```python
from build123d import *

# Parameters (mm, degrees)
F1_DEPTH  = 6
F2_R      = 27.5
F3_DEPTH  = 30
F4_R      = 14
F5_DEPTH  = 40
F6_W      = 56
F6_H      = 10
F7_DEPTH  = 8
F8_R      = 3
F9_DEPTH  = 10.5
F10_W     = 56
F10_H     = 66
F11_DEPTH = 25
F12_SIZE  = 5
F14_DEPTH = 30


with BuildPart() as f1:
    # F0 (on Front) → F1 (new body)
    with BuildSketch(Plane.XZ):
        with BuildLine():
            ThreePointArc((38, 33), (35.0710678119, 40.0710678119), (28, 43))
            Line((28, 43), (-28, 43))
            ThreePointArc((-28, 43), (-35.0710678119, 40.0710678119), (-38, 33))
            Line((-38, 33), (-38, -33))
            ThreePointArc((-38, -33), (-35.0710678119, -40.0710678119), (-28, -43))
            Line((-28, -43), (28, -43))
            ThreePointArc((28, -43), (35.0710678119, -40.0710678119), (38, -33))
            Line((38, -33), (38, 33))
        make_face()
    extrude(amount=F1_DEPTH)

    # F2 (on face) → F3 (join)
    with BuildSketch(Plane(origin=(0, 0, 0), x_dir=(-1, 0, 0), z_dir=(0, 1, 0))):
        Circle(F2_R)
    extrude(amount=F3_DEPTH)

    # F4 (on face) → F5 (join)
    with BuildSketch(Plane(origin=(0, 30, 0), x_dir=(-1, 0, 0), z_dir=(0, 1, 0))):
        Circle(F4_R)
    extrude(amount=F5_DEPTH)

    # F6 (on face) → F7 (join)
    with BuildSketch(Plane.XZ.offset(6)):
        with Locations((0, -38)):
            Rectangle(F6_W, F6_H)
    extrude(amount=F7_DEPTH)

    # F8 (on face) → F9 (join)
    with BuildSketch(Plane(origin=(0, 0, -43), x_dir=(1, 0, 0), z_dir=(0, 0, -1))):
        with Locations((-20, 10.148444213)):
            Circle(F8_R)
        with Locations((20, 10.148444213)):
            Circle(F8_R)
    extrude(amount=F9_DEPTH)

    # F10 (on face) → F11 (join)
    with BuildSketch(Plane.XZ.offset(6)):
        Rectangle(F10_W, F10_H)
    extrude(amount=F11_DEPTH)

    # F12
    f12_edges = [f1.edges().sort_by_distance(p)[0] for p in [
        (0, -31, 33),
        (28, -31, 0),
        (-28, -31, 0),
        (-28, -18.5, 33),
        (28, -18.5, 33),
        (28, -22.5, -33),
        (0, -31, -33),
        (-28, -22.5, -33),
        (0, -6, 43),
    ]]
    chamfer(f12_edges, length=F12_SIZE)

    # F13 (on face) → F14 (cut, through all)
    with BuildSketch(Plane(origin=(0, 30, 0), x_dir=(-1, 0, 0), z_dir=(0, 1, 0))):
        with BuildLine():
            Line((-17.7552809046, 21), (17.7552809046, 21))
            ThreePointArc((17.7552809046, 21), (0, 27.5), (-17.7552809046, 21))
        make_face()
        with BuildLine():
            ThreePointArc((27.5, 0), (25.8239230172, 9.4538352006), (21, 17.7552809046))
            Line((21, 17.7552809046), (21, -17.7552809046))
            ThreePointArc((21, -17.7552809046), (25.8239230172, -9.4538352006), (27.5, 0))
        make_face()
        with BuildLine():
            ThreePointArc((-17.7552809046, -21), (0, -27.5), (17.7552809046, -21))
            Line((17.7552809046, -21), (-17.7552809046, -21))
        make_face()
        with BuildLine():
            Line((-21, -17.7552809046), (-21, 17.7552809046))
            ThreePointArc((-21, 17.7552809046), (-27.5, 0), (-21, -17.7552809046))
        make_face()
    extrude(amount=-F14_DEPTH, mode=Mode.SUBTRACT)


solid = f1.part
```
Can you work these out from the model? Positions are in its coordinate system, mm. A direction names the side the tool comes from. Give positions to 0.01 mm unless a question says otherwise; leave off trailing zeros. Order: outer loops, then holes, each group sorted by start corner. A loop starts at its lowest first (then second) coordinate and runs counter-clockwise, first axis right, second up. Notation, with made-up numbers: (3, 74) - (35, 74) arc R23 ccw to (35, 108) - close; hole circle Ø3 at (42.5, 37.5). An arc over 180 degrees is marked (long way). Use a Markdown table: item, result. Add a question column.
Q1. If we mould it in two halves opening along X, with no side actions, what happens to faces 6 (the flat face through (-24.5, -27.6, -29.9)), 7 (the flat face through (25, -20, -31)), 8 (the cylindrical face through (-22.21, -12.18, -48.18)), 9 (the flat face through (0, 15, -21))? For each: released by +X, released by -X, zero draft, split by the parting line, or undercut.
Q2. If we section it at C-C on z = 15.5: Write out the boundary of the cut face in (x, y), plus the area to 3 significant figures.
Q3. If we section it at B-B on y = -19.5: Write out the boundary of the cut face in (x, z).
Q4. Please list where these lines run through material, in increasing order: line 1 along Y through (x, z) = (-27, -41); line 2 along Y through (x, z) = (-29.5, 10); line 3 along Z through (x, y) = (6.5, 15).
Q5. On a 3-axis mill with a long thin cutter (end or side, diameter ignored), from which of +Z, -Z, +X, -X, +Y, -Y can I reach the whole of each face in a straight line? I mean faces 1 (the cylindrical face through (-12.932, 49.72, -5.362)), 2 (the flat face through (25, -16, 31)), 3 (the cylindrical face through (19.47, 14.79, -19.42)), 4 (the flat face through (-25, -16, 31)), 5 (the flat face through (0, -20, -33)). Say none if no direction works.
Q6. I'm going to push flat-ended pins straight in: pin 1 (3 mm diameter, centred on x = -26.5, z = -2, fed in from -Y); pin 2 (16 mm diameter, centred on x = -3.5, y = -19, fed in from +Z); pin 3 (11 mm diameter, centred on x = -5.5, y = -10, fed in from -Z). Where does each tip first touch, or does it pass through?
Q7. If we section it at A-A on x = 0: Write out the boundary of the cut face in (y, z), plus the area to 3 significant figures.
Q8. If we section it at D-D on z = 0: Write out the boundary of the cut face in (x, y).
Answers follow:
| question | item | result |
|---|---|---|
| 1 | face 6 | released by -X |
| 1 | face 7 | released by +X |
| 1 | face 8 | undercut |
| 1 | face 9 | zero draft |
| 2 | outline | (-38, -1) - (-33, -6) - (-28, -6) - (-28, -26) - (-23, -31) - (23, -31) - (28, -26) - (28, -6) - (33, -6) - (38, -1) - (38, 0) - (21, 0) - (21, 30) - (-21, 30) - (-21, 0) - (-38, 0) - close |
| 2 | area | 3,070 mm^2 |
| 3 | outline | (-28, -28) - (-23, -33) - (23, -33) - (28, -28) - (28, 28) - (23, 33) - (-23, 33) - (-28, 28) - close |
| 4 | line 1 | y = -14 to 0 |
| 4 | line 2 | y = -6 to 0 |
| 4 | line 3 | z = -21 to 21 |
| 5 | face 1 | +Y |
| 5 | face 2 | +Z, +X, -Y |
| 5 | face 3 | -Z, +X, +Y |
| 5 | face 4 | +Z, -X, -Y |
| 5 | face 5 | -Z, +X, -X, -Y |
| 6 | pin 1 | stops at y = -29 |
| 6 | pin 2 | stops at z = 33 |
| 6 | pin 3 | stops at z = -43 |
| 7 | outline | (-31, -28) - (-26, -33) - (-14, -33) - (-14, -43) - (0, -43) - (0, -21) - (30, -21) - (30, -14) - (70, -14) - (70, 14) - (30, 14) - (30, 21) - (0, 21) - (0, 43) - (-1, 43) - (-6, 38) - (-6, 33) - (-26, 33) - (-31, 28) - close |
| 7 | area | 4,590 mm^2 |
| 8 | outline | (-38, -1) - (-33, -6) - (-28, -6) - (-28, -26) - (-23, -31) - (23, -31) - (28, -26) - (28, -6) - (33, -6) - (38, -1) - (38, 0) - (21, 0) - (21, 30) - (14, 30) - (14, 70) - (-14, 70) - (-14, 30) - (-21, 30) - (-21, 0) - (-38, 0) - close |
